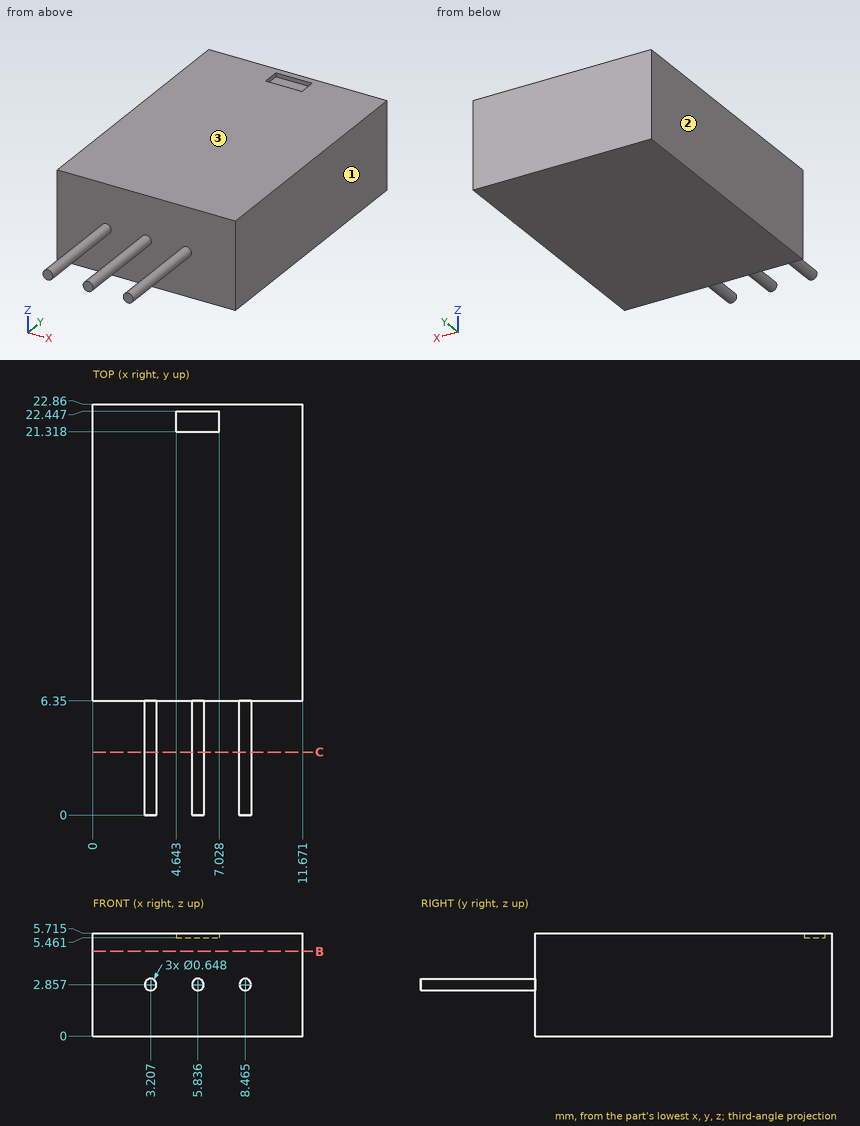
Drawing for the job (mm, zero at the part's lowest x, y, z). Give positions to 0.01 mm unless a question says otherwise; leave off trailing zeros. Order: outer loops, then holes, each group sorted by start corner. A loop starts at its lowest first (then second) coordinate and runs counter-clockwise, first axis right, second up. Notation, with made-up numbers: (88.5, 7.5) - (96.5, 7.5) arc R19 cw to (96.5, 12.5) - close; hole circle Ø5 at (-33.5, -39.75). An arc over 180 degrees is marked (long way). Use one line per item in the form item = value.
Item 1: Pin check, flat tips, straight feed: pin 1 Ø0.6 at (x, y) = (6, 21.5) entering from +Z (1 decimal); pin 2 Ø4 at (x, y) = (2.5, 3) entering from -Z. Stop position of each tip, or through.
Solution:
pin_1 = 5.7
pin_2 = 2.53
Item 2: Slice it at B-B on z = 4.7. Give the cut face in (x, y), and give its area (3 significant figures).
Solution:
outline = (0, 6.35) - (11.67, 6.35) - (11.67, 22.86) - (0, 22.86) - close
area = 193 mm2
Item 3: Probe probe 1 along X at (y, z) = (4, 2.65) (1 decimal); probe 2 along Y at (x, z) = (10, 3.7). List the from-to ranges inside material, lowest first. Write a range as from..to.
Solution:
probe_1 = 3..3.5, 5.6..6.1, 8.2..8.7
probe_2 = 6.35..22.86
Item 4: Two-plate mould, pull along X, no slides. Class the marked faces 1, 2 and 3: released by +X, released by -X, zero draft, split by the parting line, or undercut.
Solution:
face_1 = released by +X
face_2 = released by -X
face_3 = zero draft
Item 5: Slice it at C-C on y = 3.5. Give the cut face in (x, z) (1 decimal).
Solution:
outline = circle Ø0.6 at (3.2, 2.9); circle Ø0.6 at (5.8, 2.9); circle Ø0.6 at (8.5, 2.9)
